from build123d import *

# Parameters (mm, degrees)
CROQUIS1_W                 = 12
CROQUIS1_H                 = 12
SALIENTE_EXTRUIR1_DEPTH    = 36
VACIADO1_T                 = -1
CORTAR_EXTRUIR1_DEPTH      = 37.986484018
CORTAR_EXTRUIR1_DEPTH_BACK = 3
CROQUIS2_R                 = 3.25
CROQUIS3_W                 = 13.652855543
CROQUIS3_H                 = 1.6
CORTAR_EXTRUIR2_DEPTH      = 9
CROQUIS4_W                 = 10
CROQUIS4_H                 = 1
SALIENTE_EXTRUIR2_DEPTH    = 11
CROQUIS5_R                 = 2
CORTAR_EXTRUIR3_DEPTH      = 37.986484018


with BuildPart() as part:
    # Croquis1 → Saliente-Extruir1 (new body)
    with BuildSketch(Plane(origin=(0, 0, 0), x_dir=(1, 0, 0), z_dir=(0, 1, 0))):
        Rectangle(CROQUIS1_W, CROQUIS1_H)
    extrude(amount=SALIENTE_EXTRUIR1_DEPTH)

    # Vaciado1
    vaciado1_openings = [part.faces().sort_by_distance(p)[0] for p in [
        (0, 18, 6),
    ]]
    offset(amount=VACIADO1_T, openings=vaciado1_openings, kind=Kind.INTERSECTION)

    # Croquis2 → Cortar-Extruir1 (cut, two sides: drawn at the far end of the back side and taken through both)
    with BuildSketch(Plane(origin=(0, 36, 0), x_dir=(1, 0, 0), z_dir=(0, 1, 0)).offset(-CORTAR_EXTRUIR1_DEPTH_BACK)):
        with Locations(Location((0, 0, 0), (0, 0, 90))):
            Circle(CROQUIS2_R)
    extrude(amount=CORTAR_EXTRUIR1_DEPTH + CORTAR_EXTRUIR1_DEPTH_BACK, mode=Mode.SUBTRACT)

    # Croquis3 → Cortar-Extruir2 (cut)
    with BuildSketch(Plane.XY.offset(6)):
        with Locations((0.0537514, 1.8)):
            Rectangle(CROQUIS3_W, CROQUIS3_H)
    extrude(amount=-CORTAR_EXTRUIR2_DEPTH, mode=Mode.SUBTRACT)

    # Croquis4 → Saliente-Extruir2 (add)
    with BuildSketch(Plane.XY.offset(6)):
        with Locations((0, 3.1)):
            Rectangle(CROQUIS4_W, CROQUIS4_H)
    extrude(amount=-SALIENTE_EXTRUIR2_DEPTH)

    # Croquis5 → Cortar-Extruir3 (cut, through all)
    with BuildSketch(Plane(origin=(0, 36, 0), x_dir=(1, 0, 0), z_dir=(0, 1, 0))):
        with Locations(Location((0, 0, 0), (0, 0, 270))):
            Circle(CROQUIS5_R)
    extrude(amount=-CORTAR_EXTRUIR3_DEPTH, mode=Mode.SUBTRACT)


solid = part.part
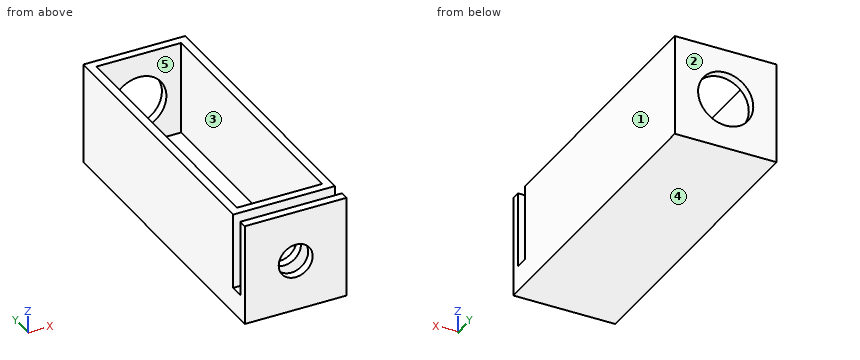
Verification items for the finished model (mm, model axes). Face numbers are marked on the shaded views. A direction names the side the tool comes from. Coordinates: 2 decimals unless noted, no trailing zeros. Write each loop counter-clockwise with the first axis right and the second up, starting at its lowest first coordinate (ties: lowest second). Pieces come first, ordered by that corner, then holes. Notation, with made-up numbers: M 36,-34 L 46,-34 A30 ccw 46,1 Z; hole C -1.75,-22 d5. An arc over 180 degrees is marked long. Use a Markdown table: item, result.
Q1. Sectioned sample at A-A, the plane z = 4.25. Record the boundary of the cut face in (x, y), plus the area to 3 significant figures.
Reply:
| item | result |
|---|---|
| outline | M -6,0 L 6,0 L 6,1 L -6,1 Z; M -6,2.6 L 6,2.6 L 6,36 L -6,36 Z; hole M -5,3.6 L 5,3.6 L 5,35 L -5,35 Z |
| area | 98.8 mm² |
Q2. Sectioned sample at C-C, the plane z = 0. Record the boundary of the cut face in (x, y).
Reply:
| item | result |
|---|---|
| outline | M -6,0 L -2,0 L -2,1 L -6,1 Z; M -6,2.6 L -2,2.6 L -2,3.6 L -5,3.6 L -5,35 L -3.25,35 L -3.25,36 L -6,36 Z; M 2,0 L 6,0 L 6,1 L 2,1 Z; M 2,2.6 L 6,2.6 L 6,36 L 3.25,36 L 3.25,35 L 5,35 L 5,3.6 L 2,3.6 Z |
Q3. Sectioned sample at B-B, the plane x = 0. Record the boundary of the cut face in (y, z).
Reply:
| item | result |
|---|---|
| outline | M 0,-6 L 36,-6 L 36,-3.25 L 35,-3.25 L 35,-5 L 3.6,-5 L 3.6,-2 L 2.6,-2 L 2.6,-5 L 1,-5 L 1,-2 L 0,-2 Z; M 0,2 L 1,2 L 1,6 L 0,6 Z; M 2.6,2 L 3.6,2 L 3.6,6 L 2.6,6 Z; M 35,3.25 L 36,3.25 L 36,6 L 35,6 Z |
Q4. Thickness scan on line 1 (Y direction, x = 0, z = 5.25); line 2 (X direction, y = 17, z = 4.5); line 3 (X direction, y = 0.2, z = 0). Record the ranges inside material, lowest first.
Reply:
| item | result |
|---|---|
| line 1 | y = 0 to 1, 2.6 to 3.6, 35 to 36 |
| line 2 | x = -6 to -5, 5 to 6 |
| line 3 | x = -6 to -2, 2 to 6 |
Q5. Set-up check for the marked faces 4 and 5: record each of +Z, -Z, +X, -X, +Y, -Y from which the full face is reachable in a straight line by a thin tool's end or side.
Reply:
| item | result |
|---|---|
| face 4 | -Z, +X, -X, +Y, -Y |
| face 5 | +Z |
Q6. Sectioned sample at D-D, the plane x = -2.5. Record the boundary of the cut face in (y, z).
Reply:
| item | result |
|---|---|
| outline | M 0,-6 L 36,-6 L 36,-2.08 L 35,-2.08 L 35,-5 L 3.6,-5 L 3.6,6 L 2.6,6 L 2.6,-5 L 1,-5 L 1,6 L 0,6 Z; M 35,2.08 L 36,2.08 L 36,6 L 35,6 Z |
Q7. Draft check along Y on the marked faces 1, 2 and 3. Enter one of: +Y half, -Y half, draft (parallel to the pull), parting line (faces both ways), or undercut.
Reply:
| item | result |
|---|---|
| face 1 | draft |
| face 2 | +Y half |
| face 3 | undercut |
Q8. Go/stop test with flat-tipped pins: P1, Ø1.1, axis at x = 5.5, y = 2, coming from the +Z side; P2, Ø3.5, axis at x = 0, z = 0, coming from the +Y side. Record where each tip stops, or that it passes through.
Reply:
| item | result |
|---|---|
| P1 | stops at z = -3 |
| P2 | passes through |
